from build123d import *

# Parameters (mm, degrees)
SKETCH_1_R               = 13
EXTRUDE_1_DEPTH          = 3.7
SKETCH_2_R               = 0.9
CUT_EXTRUDE_1_DEPTH      = 19.753399692
SKETCH_2_3_R             = 1.5
CUT_EXTRUDE_2_DEPTH      = 1.5
PATTERN_CIRCULAR_1_COUNT = 6
SKETCH_3_R               = 1.1
CUT_EXTRUDE_3_DEPTH      = 19.753399692


with BuildPart() as part:
    # Sketch 1 → Extrude 1 (new body)
    with BuildSketch(Plane.XY):
        Circle(SKETCH_1_R)
    extrude(amount=EXTRUDE_1_DEPTH)

    # Sketch 2 → Cut-Extrude 1 (cut, through all)
    with BuildSketch(Plane(origin=(0, 0, 0), x_dir=(-1, 0, 0), z_dir=(0, 0, -1))):
        with Locations((0, 8)):
            Circle(SKETCH_2_R)
    cut_extrude_1 = extrude(amount=-CUT_EXTRUDE_1_DEPTH, mode=Mode.SUBTRACT)

    # Sketch 2_3 → Cut-Extrude 2 (cut)
    with BuildSketch(Plane(origin=(0, 0, 0), x_dir=(-1, 0, 0), z_dir=(0, 0, -1))):
        with Locations((0, 8)):
            Circle(SKETCH_2_3_R)
    cut_extrude_2 = extrude(amount=-CUT_EXTRUDE_2_DEPTH, mode=Mode.SUBTRACT)

    # Pattern Circular 1: Cut-Extrude 1, Cut-Extrude 2 ×6 about axis
    pattern_circular_1_axis = Axis((0, 0, 0), (0, 0, 1))
    add([cut_extrude_1.rotate(pattern_circular_1_axis, i * 360 / PATTERN_CIRCULAR_1_COUNT) for i in range(1, PATTERN_CIRCULAR_1_COUNT)], mode=Mode.SUBTRACT)
    add([cut_extrude_2.rotate(pattern_circular_1_axis, i * 360 / PATTERN_CIRCULAR_1_COUNT) for i in range(1, PATTERN_CIRCULAR_1_COUNT)], mode=Mode.SUBTRACT)

    # Sketch 3 → Cut-Extrude 3 (cut, through all)
    with BuildSketch(Plane(origin=(0, 0, 0), x_dir=(-1, 0, 0), z_dir=(0, 0, -1))):
        Circle(SKETCH_3_R)
    extrude(amount=-CUT_EXTRUDE_3_DEPTH, mode=Mode.SUBTRACT)


solid = part.part
For this review, take the finished solid that the model builds, in its own axes (mm). A direction names the side the tool comes from. Round coordinates to 2 decimals unless told otherwise and drop trailing zeros. Order: outer loops, then holes, each group sorted by start corner. A loop starts at its lowest first (then second) coordinate and runs counter-clockwise, first axis right, second up. Notation, with made-up numbers: (42.5, 22) -> (98.5, 22) arc R24 cw to (98.5, 59) -> close; hole circle Ø7 at (64.25, 56). An arc over 180 degrees is marked (long way). Write item = value, one per line. Start each with the question number.
1) Take a section at A-A on x = 0. State the section outline as (y, z) points.
2) To check wall thickness, follow line 1 (Y direction, x = 1.25, z = 0.35); line 2 (Y direction, x = -0.25, z = 2.4); line 3 (Y direction, x = -8.25, z = 1.25). State the ranges of each line that lie inside material, in increasing order. Write a range as from..to.
3) Insertion check: pin 1 (1.1 mm diameter, centred on x = -6.93, y = 4, fed in from +Z); pin 2 (0.9 mm diameter, centred on x = 0, y = 7.5, fed in from -Z); pin 3 (1.5 mm diameter, centred on x = 4.5, z = 2.5, fed in from -Y). Each pin has a flat end and moves straight along its axis. Give the tip position at first contact, or say it passes through.
4) Take a section at C-C on z = 2.95. State the section outline as (x, y) points, plus the area to 3 significant figures.
5) The part is to be moulded in two halves that separate along X. For faces 3 (the face through (3, 0, 3.7)), 4 (the face through (0.325, 6.536, 0.74)), 5 (the face through (-10.316, -7.91, 1.824)), say which applies: +X half, -X half, draft (parallel to the pull), parting line (faces both ways), or undercut.
6) Tool access review of faces 1 (the face through (-5.54, 4.57, 0.74)), 2 (the face through (7.05, -3.11, 2.58)): name each direction out of +Z, -Z, +X, -X, +Y, -Y from which nothing blocks a thin tool from reaching the whole face with its end or side.
7) Take a section at D-D on y = -4. State the section outline as (x, z) points.
8) Take a section at B-B on y = -0.5. State the section outline as (x, z) points.
Verdict:
q1.outline = (-13, 0) -> (-9.5, 0) -> (-9.5, 1.5) -> (-8.9, 1.5) -> (-8.9, 3.7) -> (-13, 3.7) -> close; (-7.1, 1.5) -> (-6.5, 1.5) -> (-6.5, 0) -> (-1.1, 0) -> (-1.1, 3.7) -> (-7.1, 3.7) -> close; (1.1, 0) -> (6.5, 0) -> (6.5, 1.5) -> (7.1, 1.5) -> (7.1, 3.7) -> (1.1, 3.7) -> close; (8.9, 1.5) -> (9.5, 1.5) -> (9.5, 0) -> (13, 0) -> (13, 3.7) -> (8.9, 3.7) -> close
q2.line_1 = -12.94..-8.83, -7.17..7.17, 8.83..12.94
q2.line_2 = -13..-8.86, -7.14..-1.07, 1.07..7.14, 8.86..13
q2.line_3 = -10.05..-4.71, -3.29..3.29, 4.71..10.05
q3.pin_1 = through
q3.pin_2 = 1.5
q3.pin_3 = -12.45
q4.outline = circle Ø26 at (0, 0); hole circle Ø1.8 at (-6.93, -4); hole circle Ø1.8 at (-6.93, 4); hole circle Ø2.2 at (0, 0); hole circle Ø1.8 at (0, -8); hole circle Ø1.8 at (0, 8); hole circle Ø1.8 at (6.93, -4); hole circle Ø1.8 at (6.93, 4)
q4.area = 512 mm2
q5.face_3 = draft
q5.face_4 = undercut
q5.face_5 = parting line
q6.face_1 = -Z
q6.face_2 = +Z, -Z
q7.outline = (-12.37, 0) -> (-8.43, 0) -> (-8.43, 1.5) -> (-7.83, 1.5) -> (-7.83, 3.7) -> (-12.37, 3.7) -> close; (-6.03, 1.5) -> (-5.43, 1.5) -> (-5.43, 0) -> (5.43, 0) -> (5.43, 1.5) -> (6.03, 1.5) -> (6.03, 3.7) -> (-6.03, 3.7) -> close; (7.83, 1.5) -> (8.43, 1.5) -> (8.43, 0) -> (12.37, 0) -> (12.37, 3.7) -> (7.83, 3.7) -> close
q8.outline = (-12.99, 0) -> (-0.98, 0) -> (-0.98, 3.7) -> (-12.99, 3.7) -> close; (0.98, 0) -> (12.99, 0) -> (12.99, 3.7) -> (0.98, 3.7) -> close
